```python
from build123d import *

# Parameters (mm, degrees)
BOSS_EXTRUDE1_DEPTH   = 2
BOSS_EXTRUDE2_DEPTH   = 5
FILLET1_R             = 3
F_1_5MM_DOWEL_HOLE1_D = 1.5


with BuildPart() as part:
    # Sketch1 → Boss-Extrude1 (new body)
    with BuildSketch(Plane.XY):
        with BuildLine():
            Line((-1.686437718, 8.505953435), (-4.658536585, -3.56097561))
            Line((-4.658536585, -3.56097561), (4.658536585, -3.56097561))
            Line((4.658536585, -3.56097561), (1.686437718, 8.505953435))
            ThreePointArc((1.686437718, 8.505953435), (0, 10.192391153), (-1.686437718, 8.505953435))
        make_face()
    extrude(amount=BOSS_EXTRUDE1_DEPTH)

    # Sketch2 → Boss-Extrude2 (add)
    with BuildSketch(Plane(origin=(0, 0, 0), x_dir=(-1, 0, 0), z_dir=(0, 0, -1))):
        Polygon((-4.450149656, -2.714910119), (4.450149656, -2.714910119), (4.658536585, -3.56097561), (-4.658536585, -3.56097561), align=None)
    extrude(amount=BOSS_EXTRUDE2_DEPTH)

    # Fillet1
    fillet1_edges = [part.edges().sort_by_distance(p)[0] for p in [
        (0, -2.714910119, 0),
    ]]
    fillet(fillet1_edges, radius=FILLET1_R)

    # Ø1.5mm Dowel Hole1 (through all)
    with Locations(Plane.XY.offset(2)):
        with Locations((0, 8.505953435), (0, 2.123465087)):
            Hole(F_1_5MM_DOWEL_HOLE1_D / 2)


solid = part.part
```
CAD build for the part. Positions are in the model's coordinates, mm. A direction names the side the tool comes from. Round coordinates to 2 decimals unless told otherwise and drop trailing zeros. Write each loop counter-clockwise with the first axis right and the second up, starting at its lowest first coordinate (ties: lowest second). Pieces come first, ordered by that corner, then holes. Notation, with made-up numbers: (-10, 79.5) - (28, 79.5) arc R21 cw to (28, 103.5) - close; hole circle Ø7 at (43, -1.5). An arc over 180 degrees is marked (long way). Write item = value, one per line. Start each with the question number.
Q1. Band-saw the part on D-D (y = 4.5). Give the cut face in (x, z), then the cut area to 3 significant figures.
Q2. Drop flat-ended pins along their axis: pin 1 (1.5 mm diameter, centred on x = -0.5, z = -3, fed in from +Y); pin 2 (2 mm diameter, centred on x = 0, y = 8.51, fed in from -Z); pin 3 (1.5 mm diameter, centred on y = -1.5, z = 0.5, fed in from +X); pin 4 (3 mm diameter, centred on x = -3, y = 7.5, fed in from +Z). Give the stop position or say it passes through.
Q3. Band-saw the part on C-C (z = -3.75). Give the cut face in (x, y), then the cut area to 3 significant figures.
Q4. Probe L1, parallel to Y at x = 0, z = 0.7; L2, parallel to Y at x = 2.5, z = -4.5; L3, parallel to Z at x = 2, y = 1.75. List the from-to ranges inside material, lowest first. Write a range as from..to.
Q5. Band-saw the part on B-B (x = 4.25). Give the cut face in (y, z), then the cut area to 3 significant figures.
Q6. Which spindle directions (+Z, -Z, +X, -X, +Y, -Y) get a long thin tool onto all of the face, cutting with end or side? Do faces 1 (the flat face through (0, -3.561, -1)), 2 (the flat face through (0, 4, 0)). Say none if no direction does.
Q7. Band-saw the part on A-A (x = 0). Give the cut face in (y, z).
Answers below:
q1.outline = (-2.67, 0) - (2.67, 0) - (2.67, 2) - (-2.67, 2) - close
q1.area = 10.7 mm2
q2.pin_1 = -2.62
q2.pin_2 = 0
q2.pin_3 = 4.34
q2.pin_4 = 2
q3.outline = (-4.66, -3.56) - (4.66, -3.56) - (4.45, -2.71) - (-4.45, -2.71) - close
q3.area = 7.71 mm2
q4.L1 = -3.56..1.37, 2.87..7.76, 9.26..10.19
q4.L2 = -3.56..-2.71
q4.L3 = 0..2
q5.outline = (-3.56, -5) - (-2.71, -5) - (-2.71, -3) arc R3 cw to (-1.9, -0.95) - (-1.9, 2) - (-3.56, 2) - close
q5.area = 8.84 mm2
q6.face_1 = +Z, -Z, +X, -X, -Y
q6.face_2 = -Z, +X, -X, +Y
q7.outline = (-3.56, -5) - (-2.71, -5) - (-2.71, -3) arc R3 cw to (0.29, 0) - (1.37, 0) - (1.37, 2) - (-3.56, 2) - close; (2.87, 0) - (7.76, 0) - (7.76, 2) - (2.87, 2) - close; (9.26, 0) - (10.19, 0) - (10.19, 2) - (9.26, 2) - close
